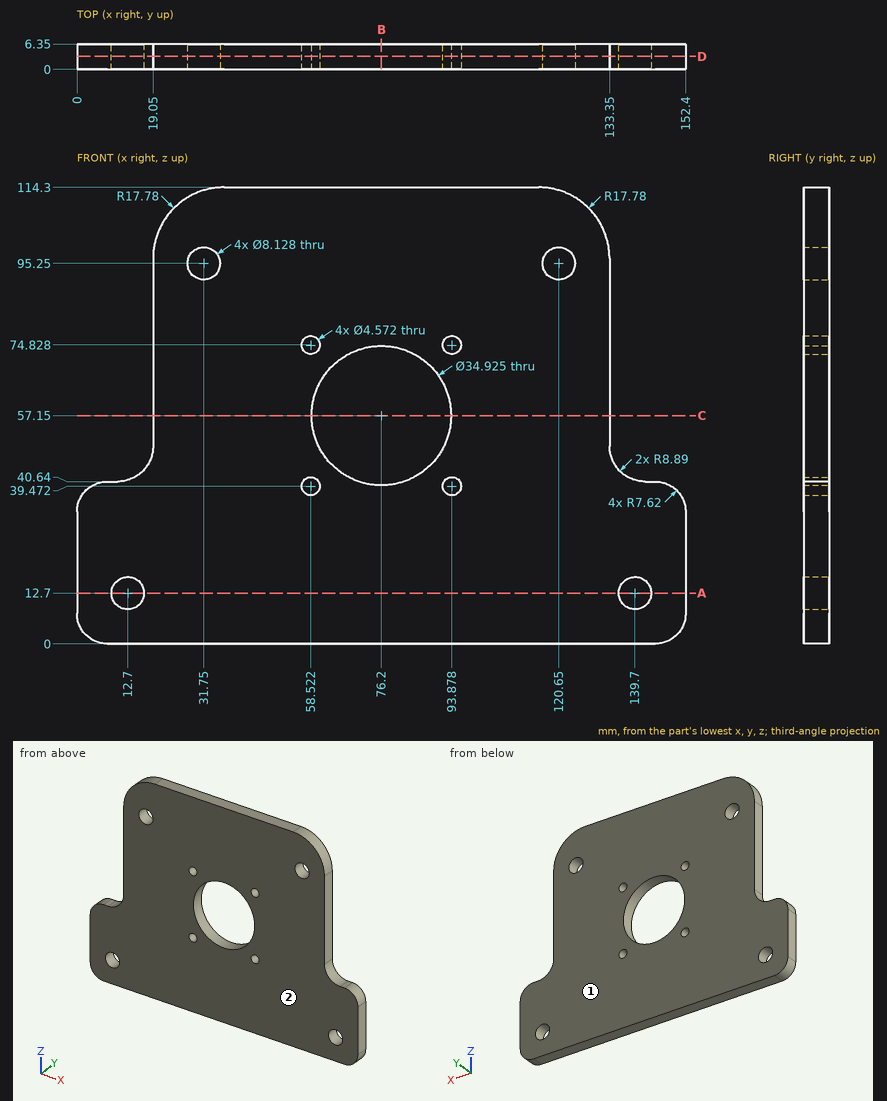
For this review, use the dimensioned drawing (mm, ordinates from the lowest corner) and the shaded views. Give positions to 0.01 mm unless a question says otherwise; leave off trailing zeros. Write each loop counter-clockwise with the first axis right and the second up, starting at its lowest first coordinate (ties: lowest second). Pieces come first, ordered by that corner, then holes. Notation, with made-up numbers: M 40,23 L 84,23 A12 cw 84,40 Z; hole C 19.5,83 d6. An arc over 180 degrees is marked long. Answer as a JSON object with one key per item and string values. Group by question number.
Item 1: For pin 1 Ø3 at (x, y) = (130, 2) entering from +Z (1 decimal); pin 2 Ø2 at (x, y) = (143.5, 4) entering from +Z; pin 3 Ø1 at (y, z) = (1.5, 93) entering from +X, all flat-tipped, find the tip position at first contact; note any pin that passes through.
Item 2: Consider section D-D on y = 3.25. Count the separate pieces of the cut face and the enclosed holes in it, plus the area to 3 significant figures.
Item 3: Draft analysis for pull direction Y (two halves, no side actions). For the marked faces 1 and 2, state which applies: +Y half, -Y half, draft (parallel to the pull), parting line (faces both ways), or undercut.
Item 4: Consider section B-B on x = 76.2. Write out the cut boundary in (y, z).
Item 5: Consider section C-C on z = 57.15. Write out the cut boundary in (x, y).
Item 6: For probe 1 along X at (y, z) = (1.75, 12.7); probe 2 along X at (y, z) = (1.5, 58); probe 3 along Z at (x, y) = (87.5, 1.25) (1 decimal), list the stretches that pass through material, from the lowest coordinate up. Write a range as [from, to].
Item 7: Consider section A-A on z = 12.7. Write out the cut boundary in (x, y).
Check result:
{
 "1": {"pin 1": "stops at z = 108.7", "pin 2": "stops at z = 40.64", "pin 3": "stops at x = 133.35"},
 "2": {"separate pieces": "1", "enclosed holes": "9", "area": "13,200 mm^2"},
 "3": {"face 1": "+Y half", "face 2": "-Y half"},
 "4": {"outline": "M 0,0 L 6.35,0 L 6.35,39.69 L 0,39.69 Z; M 0,74.61 L 6.35,74.61 L 6.35,114.3 L 0,114.3 Z"},
 "5": {"outline": "M 19.05,0 L 58.74,0 L 58.74,6.35 L 19.05,6.35 Z; M 93.66,0 L 133.35,0 L 133.35,6.35 L 93.66,6.35 Z"},
 "6": {"probe 1": "x = [0, 8.64], [16.76, 135.64], [143.76, 152.4]", "probe 2": "x = [19.05, 58.76], [93.64, 133.35]", "probe 3": "z = [0, 43.8], [70.5, 114.3]"},
 "7": {"outline": "M 0,0 L 8.64,0 L 8.64,6.35 L 0,6.35 Z; M 16.76,0 L 135.64,0 L 135.64,6.35 L 16.76,6.35 Z; M 143.76,0 L 152.4,0 L 152.4,6.35 L 143.76,6.35 Z"}
}
